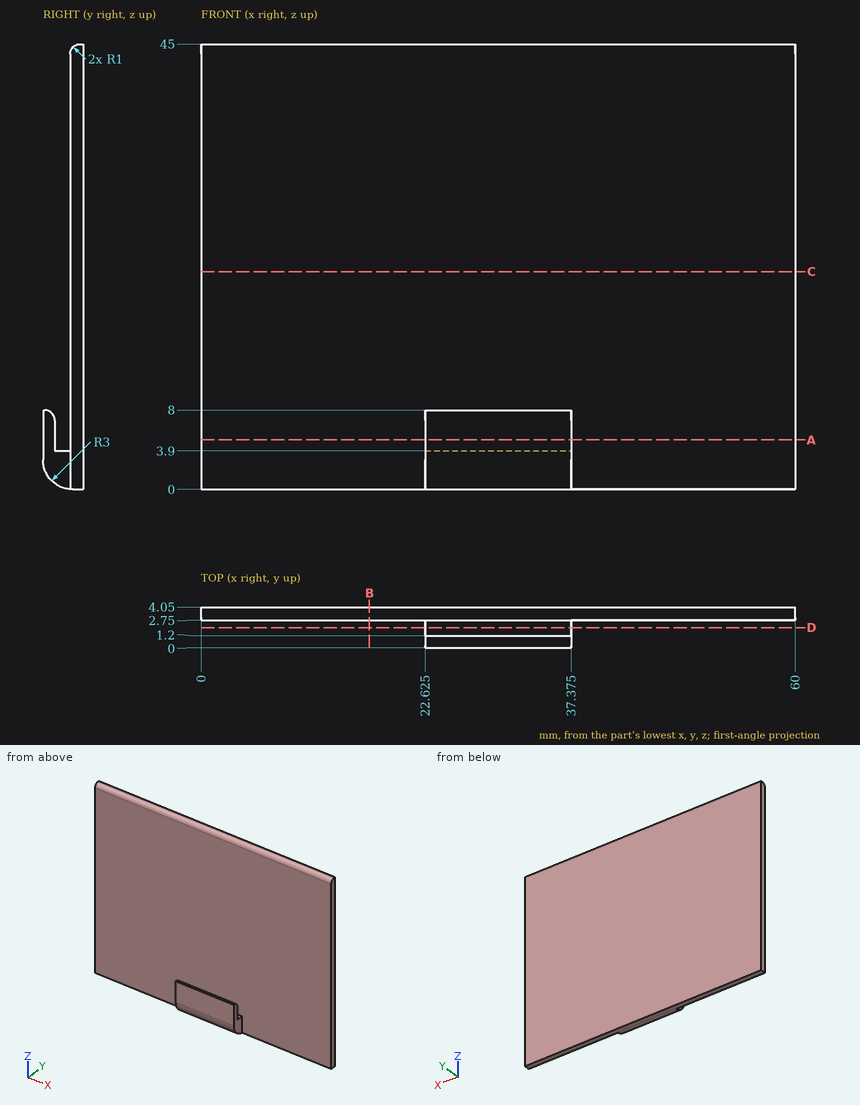
Geometry check sheet. Reference: drawing and pictorial views, mm from the part's lowest x, y, z. Round coordinates to 2 decimals unless told otherwise and drop trailing zeros. Order: outer loops, then holes, each group sorted by start corner. A loop starts at its lowest first (then second) coordinate and runs counter-clockwise, first axis right, second up.
Q1. Cross-section at A-A, the plane z = 5. Enter the section's corners in (x, y) (3 decimals).
Filled sheet:
outline: (0, 2.75) - (60, 2.75) - (60, 4.05) - (0, 4.05) - close; (22.625, 0) - (37.375, 0) - (37.375, 1.2) - (22.625, 1.2) - close
Q2. Cross-section at B-B, the plane x = 17. Enter the section's corners in (y, z), plus the area to 3 significant figures.
Filled sheet:
outline: (2.75, 0.01) arc R3 ccw to (3, 0) - (4.05, 0) - (4.05, 45) - (3.75, 45) arc R1 ccw to (2.75, 44) - close
area: 58.3 mm2
Q3. Cross-section at D-D, the plane y = 2. Enter the section's corners in (x, z) (3 decimals), plus the area to 3 significant figures.
Filled sheet:
outline: (22.625, 0.172) - (37.375, 0.172) - (37.375, 3.9) - (22.625, 3.9) - close
area: 55.0 mm2
Q4. Scan lines: L1, parallel to Y at x = 16, z = 19.5; L2, parallel to Z at x = 57, y = 3.2; L3, parallel to Z at x = 25.5, y = 1.1. Record each from-to range of solid material in increasing order.
Filled sheet:
L1: y = 2.75 to 4.05
L2: z = 0 to 44.84
L3: z = 0.68 to 7.44
Q5. Cross-section at C-C, the plane z = 22. Enter the section's corners in (x, y).
Filled sheet:
outline: (0, 2.75) - (60, 2.75) - (60, 4.05) - (0, 4.05) - close
Q6. Depth check by flat-ended pin: P1, Ø5, axis at x = 18, z = 10, coming from the -Y side; P2, Ø0.8, axis at x = 29.5, y = 2, coming from the +Z side; P3, Ø0.8, axis at y = 1, z = 3.5, coming from the +X side (3 decimals); P4, Ø2, axis at y = 2, z = 35, coming from the -X side. Enter the tip coordinate at first touch or a pass-through.
Filled sheet:
P1: stops at y = 2.75
P2: stops at z = 3.9
P3: stops at x = 37.375
P4: stops at x = 0
